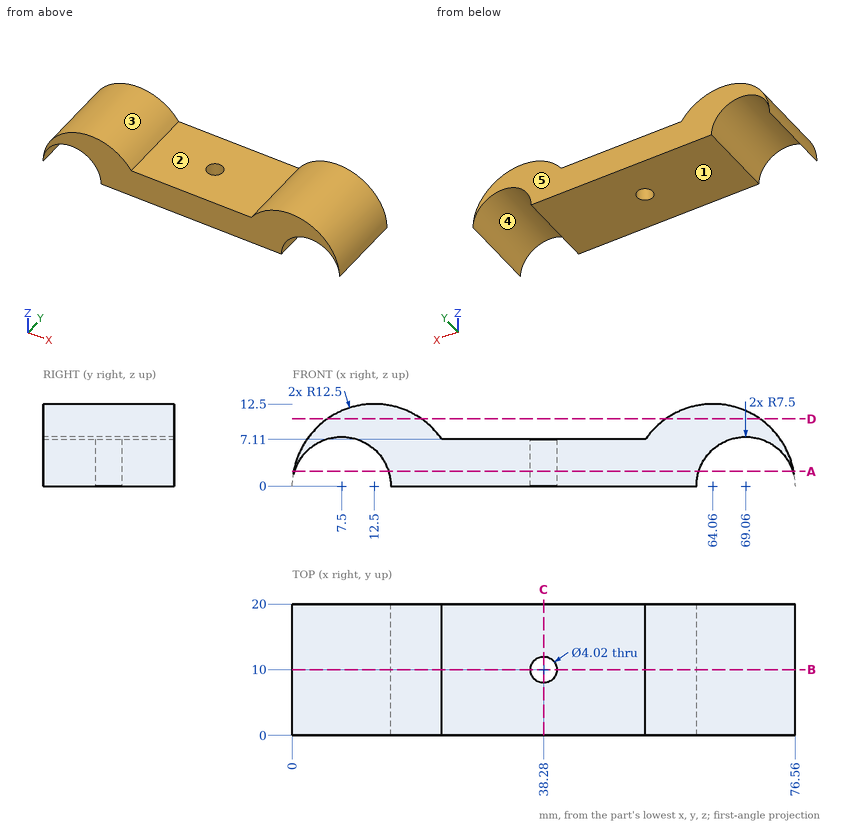
Verification items for this drawing (mm, ordinates from the low corner). A direction names the side the tool comes from. Give positions to 0.01 mm unless a question says otherwise; leave off trailing zeros. Loops run counter-clockwise (first coordinate to the right, second up) from the corner with the lowest first, then second, coordinate; pieces in that order, holes last. Notation, with made-up numbers: M -23,-9 L 3,-9 A18 ccw 3,-2 Z; hole C 9.5,83.25 d7. An arc over 180 degrees is marked long. Write item = value, one per line.
(1) Sectioned sample at D-D, the plane z = 10.25. Record the cut outline in (x, y).
Answer below:
outline = M 5.35,0 L 19.65,0 L 19.65,20 L 5.35,20 Z; M 56.91,0 L 71.21,0 L 71.21,20 L 56.91,20 Z
(2) Release check for a two-part mould opening along X. For the marked faces 3, 4 and 5 record: released by +X, released by -X, zero draft, split by the parting line, or undercut.
Answer below:
face_3 = undercut
face_4 = undercut
face_5 = zero draft
(3) Sectioned sample at C-C, the plane x = 38.28. Record the cut outline in (y, z).
Answer below:
outline = M 0,0 L 7.99,0 L 7.99,7.11 L 0,7.11 Z; M 12.01,0 L 20,0 L 20,7.11 L 12.01,7.11 Z
(4) Tool access check on the marked faces 1 and 2. Record the directions out of +Z, -Z, +X, -X, +Y, -Y that give a thin tool (end or side, any length) a straight path to the whole face; none if there is none.
Answer below:
face_1 = -Z, +X, -X, +Y, -Y
face_2 = +Z, +Y, -Y
(5) Sectioned sample at A-A, the plane z = 2.25. Record the cut outline in (x, y), plus the area to 3 significant figures.
Answer below:
outline = M 0.2,0 L 0.35,0 L 0.35,20 L 0.2,20 Z; M 14.65,0 L 61.91,0 L 61.91,20 L 14.65,20 Z; M 76.21,0 L 76.36,0 L 76.36,20 L 76.21,20 Z; hole C 38.28,10 d4.02
area = 938 mm2
(6) Sectioned sample at B-B, the plane y = 10. Record the cut outline in (x, z), plus the area to 3 significant figures.
Answer below:
outline = M 0,0 A7.5 cw 15,0 L 36.27,0 L 36.27,7.11 L 22.78,7.11 A12.5 ccw Z; M 40.29,0 L 61.56,0 A7.5 cw 76.56,0 A12.5 ccw 53.78,7.11 L 40.29,7.11 Z
area = 485 mm2
(7) Material ranges on line 1 (Y direction, x = 38.28, z = 3.5); line 2 (X direction, y = 8.5, z = 4.5); line 3 (Z direction, x = 25, y = 9.75), recorded low to high. Write a range as [from, to].
Answer below:
line_1 = [0, 7.99], [12.01, 20]
line_2 = [0.84, 1.5], [13.5, 36.94], [39.62, 63.06], [75.06, 75.72]
line_3 = [0, 7.11]
(8) Gauge pin test, flat ends, axial feed: pin 1 Ø6.5 at (x, y) = (38.28, 10) entering from +Z; pin 2 Ø5 at (y, z) = (11.5, 10.5) entering from +X; pin 3 Ø5 at (y, z) = (6.5, 7) entering from +X. Record the tip position at first contact, or that the pin passes through.
Answer below:
pin_1 = 7.11
pin_2 = 73.66
pin_3 = 75.72
